Autodesk Inventor part; units mm, degrees
ref_plane "Work Plane1" through (19.05, 73.7803, 37.8333) normal (0, 1, 0) x (-1, 0, 0)
ref_plane "YZ Plane" through (0, 0, 0) normal (1, 0, 0) x (0, 1, 0)
ref_plane "XY Plane" through (0, 0, 0) normal (0, 0, 1) x (1, 0, 0)
sketch "Sketch1" plane through (0, 0, 0) normal (0, 0, 1) x (1, 0, 0)
  arc A0 (19.05, 73.7803) -> (-19.05, 73.7803) centre (0, 0) ccw
  line L0 (0, 86.4803) -> (19.05, 86.4803)
  line L1 (19.05, 86.4803) -> (19.05, 73.7803)
  line L2 (0, 76.2) -> (0, 86.4803) construction
  line L3 (0, 86.4803) -> (-19.05, 86.4803)
  line L4 (-19.05, 86.4803) -> (-19.05, 73.7803)
  dimension "d0" = 152.4
  dimension "d1" = 19.05
  dimension "d2" = 12.7
extrude "Extrusion1" add sketch "Sketch1" along normal mid plane 75.6666
sketch "Sketch2" plane through (-19.05, 86.4803, 37.8333) normal (0, 1, 0) x (1, 0, 0)
  line L0 (0, 75.6666) -> (0, 0) construction
  line L1 (0, 37.8333) -> (38.1, 37.8333) construction
  line L2 (38.1, 75.6666) -> (38.1, 0) construction
  line L3 (0, 75.6666) -> (38.1, 75.6666) construction
  line L4 (19.05, 75.6666) -> (19.05, 0) construction
  line L5 (38.1, 0) -> (0, 0) construction
  line L6 (28.575, 32.4358) -> (28.575, 43.2308) construction
  line L7 (26.3525, 32.4358) -> (26.3525, 43.2308)
  line L8 (30.7975, 43.2308) -> (30.7975, 32.4358)
  arc A0 (26.3525, 32.4358) -> (30.7975, 32.4358) centre (28.575, 32.4358) ccw
  arc A1 (30.7975, 43.2308) -> (26.3525, 43.2308) centre (28.575, 43.2308) ccw
  line L9 (11.7475, 32.4358) -> (11.7475, 43.2308)
  line L10 (7.3025, 43.2308) -> (7.3025, 32.4358)
  arc A2 (7.3025, 32.4358) -> (11.7475, 32.4358) centre (9.525, 32.4358) ccw
  arc A3 (11.7475, 43.2308) -> (7.3025, 43.2308) centre (9.525, 43.2308) ccw
  point P0 (19.05, 37.8333)
  point P1 (28.575, 37.8333)
  dimension "d5" = 9.525
  dimension "d6" = 4.445
  dimension "d7" = 15.24
  dimension "d8" = 19.05
extrude "Extrusion2" cut sketch "Sketch2" against normal through all
ref_plane "Work Plane1" through (19.05, 73.7803, 37.8333) normal (0, 1, 0) x (-1, 0, 0)
sketch "Sketch4" plane through (19.05, 73.7803, 37.8333) normal (0, 1, 0) x (-1, 0, 0)
  line L0 (11.7475, -43.2308) -> (11.7475, -32.4358)
  line L1 (11.7475, -32.4358) -> (11.7475, -43.2308) construction
  line L2 (11.7475, -37.8333) -> (7.3025, -37.8333) construction
  line L3 (7.3025, -43.2308) -> (7.3025, -32.4358) construction
  line L4 (9.525, -41.6433) -> (9.525, -34.0233) construction
  line L5 (15.24, -41.6433) -> (15.24, -34.0233)
  line L6 (3.81, -34.0233) -> (3.81, -41.6433)
  arc A0 (3.81, -41.6433) -> (15.24, -41.6433) centre (9.525, -41.6433) ccw
  arc A1 (15.24, -34.0233) -> (3.81, -34.0233) centre (9.525, -34.0233) ccw
  line L7 (0, 0) -> (38.1, 0) construction
  line L8 (19.05, 0) -> (19.05, -75.6666) construction
  line L9 (38.1, -75.6666) -> (0, -75.6666) construction
  line L10 (22.86, -41.6433) -> (22.86, -34.0233)
  line L11 (34.29, -34.0233) -> (34.29, -41.6433)
  arc A2 (22.86, -41.6433) -> (34.29, -41.6433) centre (28.575, -41.6433) ccw
  arc A3 (34.29, -34.0233) -> (22.86, -34.0233) centre (28.575, -34.0233) ccw
  point P0 (19.05, -37.8333)
  point P1 (9.525, -37.8333)
  dimension "d11" = 11.43
  dimension "d12" = 19.05
extrude "Extrusion3" cut sketch "Sketch4" along normal blind 7.62
sketch "Sketch20" plane through (19.05, 73.7803, 37.8333) normal (1, 0, 0) x (0, 0, -1)
  line L0 (0, 12.7) -> (0, 0)
  line L1 (75.6666, 12.7) -> (0, 12.7)
  line L2 (0, 6.35) -> (75.6666, 6.35)
  line L3 (75.6666, 6.35) -> (75.6666, 12.7)
  line L4 (75.6666, 12.7) -> (0, 12.7)
  line L5 (0, 12.7) -> (0, 6.35)
  point P0 (37.8333, -73.7803)
extrude "Extrusion7" cut sketch "Sketch20" against normal through all
sketch "Sketch21" plane through (19.05, 80.1303, 37.8333) normal (0, 1, 0) x (1, 0, 0)
  line L0 (-38.1, 75.6666) -> (0, 75.6666) construction
  line L1 (0, 0) -> (-38.1, 0) construction
  point P0 (-19.05, 37.8333)
  point P1 (-19.05, 59.7916)
  point P2 (-19.05, 15.875)
  dimension "d170" = 15.875
  dimension "d171" = 15.875
hole "Hole1" at (0, 80.1303, -21.9583) at (0, 80.1303, 21.9583) direction (0, -1, 0) diameter 3.9624 end through all
equation "\"d51\" = 0.125 * Sketch8_Pitch"
equation "\"Sketch8_Pitch\" = 0.79375"
equation "\"d53\" = 60deg"
equation "\"d72\" = 0.125 * Sketch10_Pitch"
equation "\"Sketch10_Pitch\" = 0.79375"
equation "\"d74\" = 60deg"
equation "\"d93\" = 0.125 * Sketch12_Pitch"
equation "\"Sketch12_Pitch\" = 0.79375"
equation "\"d95\" = 60deg"
equation "\"d114\" = 0.125 * Sketch14_Pitch"
equation "\"Sketch14_Pitch\" = 0.79375"
equation "\"d116\" = 60deg"
equation "\"d135\" = 0.125 * Sketch16_Pitch"
equation "\"Sketch16_Pitch\" = 0.79375"
equation "\"d137\" = 60deg"
equation "\"d156\" = 0.125 * Sketch18_Pitch"
equation "\"Sketch18_Pitch\" = 0.79375"
equation "\"d158\" = 60deg"
properties part number "finderSupportPartV05"
Check sheet for the modelled part. Datum: model origin and axes. Units: mm. A direction names the side the tool comes from. Give positions to 0.01 mm unless a question says otherwise; leave off trailing zeros. Loops run counter-clockwise (first coordinate to the right, second up) from the corner with the lowest first, then second, coordinate; pieces in that order, holes last. Notation, with made-up numbers: M 41.25,50.25 L 84.25,50.25 A32 ccw 84.25,89.25 Z; hole C 77.25,29.25 d2. An arc over 180 degrees is marked long. Use a Markdown table: item, result. Add a question column.
Q1. Tool access check on faces 5 (the flat face through (19.05, 77, -1)), 6 (the cylindrical face through (9.399, 77.965, -9.524)). Record the directions out of +Z, -Z, +X, -X, +Y, -Y that give a thin tool (end or side, any length) a straight path to the whole face; none if there is none.
Q2. Scan lines: line 1 along Z through (x, y) = (0, 77.55); line 2 along X through (y, z) = (79.5, -22); line 3 along X through (y, z) = (78.75, -6.5). Record each from-to range of solid material in increasing order. Write a range as [from, to].
Q3. Go/stop test with a flat-tipped pin: pin 1 (6.5 mm diameter, centred on x = 0, z = 21.96, fed in from -Y). Record where the tip stops, or that it passes through.
Q4. Sectioned sample at C-C, the plane x = 14.5. Record the cut outline in (y, z).
Q5. Sectioned sample at D-D, the plane z = 5. Record the cut outline in (x, y).
Q6. Sectioned sample at B-B, the plane y = 78.5. Give the number of separate pieces and of enclosed holes in the cut face, then the cut area to 3 significant figures.
Q7. Mould release check, pull along Z, two halves, no side actions. Record for faces 1 (the flat face through (0, 78, 37.833)), 2 (the flat face through (-15.24, 77, 0)), 3 (the flat face through (15.24, 77, 0)), 4 (the flat face through (-19.05, 77, -1)): pulls with the +Z half, pulls with the -Z half, needs draft (parallel to the pull), parting line crosses it, or undercut.
Q8. Sectioned sample at A-A, the plane x = 0. Record the cut outline in (y, z), then the cut area to 3 significant figures.
Verdict:
| question | item | result |
|---|---|---|
| 1 | face 5 | +Z, -Z, +X, +Y, -Y |
| 1 | face 6 | +Y, -Y |
| 2 | line 1 | [-37.83, -23.94], [-19.98, 19.98], [23.94, 37.83] |
| 2 | line 2 | [-19.05, -1.98], [1.98, 19.05] |
| 2 | line 3 | [-19.05, -14.57], [-4.48, 4.48], [14.57, 19.05] |
| 3 | pin 1 | y = 76.13 |
| 4 | outline | M 74.81,-37.83 L 80.13,-37.83 L 80.13,-6.62 L 74.81,-6.62 Z; M 74.81,6.62 L 80.13,6.62 L 80.13,37.83 L 74.81,37.83 Z |
| 5 | outline | M -19.05,73.78 A76.2 cw -15.11,74.69 L -15.11,80.13 L -19.05,80.13 Z; M -3.94,76.1 A76.2 cw 3.94,76.1 L 3.94,80.13 L -3.94,80.13 Z; M 15.11,74.69 A76.2 cw 19.05,73.78 L 19.05,80.13 L 15.11,80.13 Z |
| 6 | separate pieces | 1 |
| 6 | enclosed holes | 4 |
| 6 | area | 2,480 mm^2 |
| 7 | face 1 | pulls with the +Z half |
| 7 | face 2 | undercut |
| 7 | face 3 | undercut |
| 7 | face 4 | needs draft |
| 8 | outline | M 76.2,-37.83 L 80.13,-37.83 L 80.13,-23.94 L 76.2,-23.94 Z; M 76.2,-19.98 L 80.13,-19.98 L 80.13,19.98 L 76.2,19.98 Z; M 76.2,23.94 L 80.13,23.94 L 80.13,37.83 L 76.2,37.83 Z |
| 8 | area | 266 mm^2 |
